from build123d import *

# Parameters (mm, degrees)
EXTRUDE_1_DEPTH     = 4
SKETCH_3_R          = 1.525
CUT_EXTRUDE_3_DEPTH = 5
SKETCH_6_R          = 9.5
CUT_EXTRUDE_5_DEPTH = 5
FILLET_1_R          = 3
SKETCH_7_R          = 1.525
CUT_EXTRUDE_6_DEPTH = 10
CUT_EXTRUDE_7_DEPTH = 10
FILLET_2_R          = 1


with BuildPart() as part:
    # 草图1 → 凸台-拉伸1 (new body)
    with BuildSketch(Plane(origin=(0, 0, 0), x_dir=(1, 0, 0), z_dir=(0, 1, 0))):
        with BuildLine():
            ThreePointArc((-22.5, 20), (-42.5, 0), (-22.5, -20))
            Line((-22.5, -20), (-22.5, 20))
        make_face()
        with BuildLine():
            Line((-22.5, 20), (-22.5, -20))
            ThreePointArc((-22.5, -20), (-8.357864376, -14.142135624), (-2.5, 0))
            ThreePointArc((-2.5, 0), (-8.357864376, 14.142135624), (-22.5, 20))
        make_face()
        with BuildLine():
            ThreePointArc((-2.5, 0), (-8.357864376, -14.142135624), (-22.5, -20))
            Line((-22.5, -20), (22.5, -20))
            Line((22.5, -20), (22.5, 20))
            Line((22.5, 20), (-22.5, 20))
            ThreePointArc((-22.5, 20), (-8.357864376, 14.142135624), (-2.5, 0))
        make_face()
    extrude(amount=EXTRUDE_1_DEPTH)

    # 草图3 → 切除-拉伸3 (cut, through all)
    with BuildSketch(Plane(origin=(0, 0, 0), x_dir=(1, 0, 0), z_dir=(0, 1, 0))):
        with Locations((-36, 0)):
            Circle(SKETCH_3_R)
        with Locations((-29.25, 11.691342951)):
            Circle(SKETCH_3_R)
        with Locations((-15.75, 11.691342951)):
            Circle(SKETCH_3_R)
        with Locations((-9, 0)):
            Circle(SKETCH_3_R)
        with Locations((-15.75, -11.691342951)):
            Circle(SKETCH_3_R)
        with Locations((-29.25, -11.691342951)):
            Circle(SKETCH_3_R)
    extrude(amount=CUT_EXTRUDE_3_DEPTH, mode=Mode.SUBTRACT)

    # 草图6 → 切除-拉伸5 (cut, through all)
    with BuildSketch(Plane.XZ):
        with Locations((-22.5, 0)):
            Circle(SKETCH_6_R)
    extrude(amount=-CUT_EXTRUDE_5_DEPTH, mode=Mode.SUBTRACT)

    # 圆角1
    fillet_1_edges = [part.edges().sort_by_distance(p)[0] for p in [
        (22.5, 2, -20),
        (22.5, 2, 20),
    ]]
    fillet(fillet_1_edges, radius=FILLET_1_R)

    # 草图7 → 切除-拉伸6 (cut)
    with BuildSketch(Plane(origin=(0, 4, 0), x_dir=(1, 0, 0), z_dir=(0, 1, 0))):
        with Locations((19, -14)):
            Circle(SKETCH_7_R)
        with Locations((18.999999998, 13.999999998)):
            Circle(SKETCH_7_R)
    extrude(amount=-CUT_EXTRUDE_6_DEPTH, mode=Mode.SUBTRACT)

    # 草图8 → 切除-拉伸7 (cut)
    with BuildSketch(Plane.XZ):
        with BuildLine():
            Line((-2.5, 4), (12.5, 4))
            Line((12.5, 4), (12.5, 12))
            Line((12.5, 12), (0.5, 12))
            ThreePointArc((0.5, 12), (-0.274661673, 7.727998127), (-2.5, 4))
        make_face()
        with BuildLine():
            Line((12.5, -12), (0.5, -12))
            ThreePointArc((0.5, -12), (-0.274661673, -7.727998127), (-2.5, -4))
            Line((-2.5, -4), (12.5, -4))
            Line((12.5, -4), (12.5, -12))
        make_face()
    extrude(amount=-CUT_EXTRUDE_7_DEPTH, mode=Mode.SUBTRACT)

    # 圆角2
    fillet_2_edges = [part.edges().sort_by_distance(p)[0] for p in [
        (-2.5, 2, 4),
        (0.5, 2, 12),
        (12.5, 2, 12),
        (12.5, 2, 4),
        (0.5, 2, -12),
        (-2.5, 2, -4),
        (12.5, 2, -4),
        (12.5, 2, -12),
    ]]
    fillet(fillet_2_edges, radius=FILLET_2_R)


solid = part.part
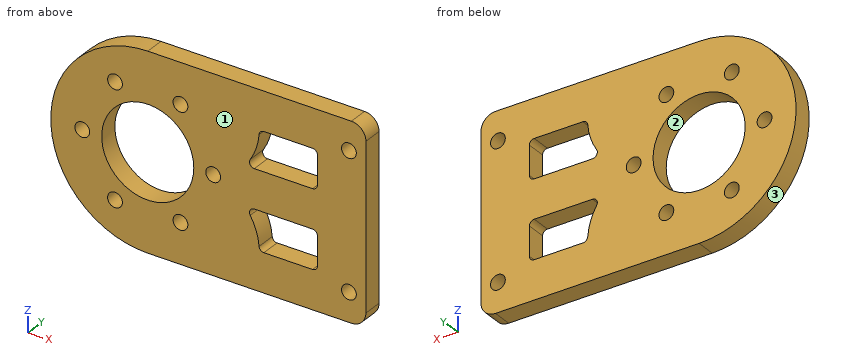
Here's how the part is built. I have some questions about the finished solid (model axes, mm). Face numbers are marked on the shaded views. Give positions to 0.01 mm unless a question says otherwise; leave off trailing zeros. Order: outer loops, then holes, each group sorted by start corner. A loop starts at its lowest first (then second) coordinate and runs counter-clockwise, first axis right, second up. Notation, with made-up numbers: M 57,-11 L 69,-11 A18 cw 69,20 Z; hole C 11,42.25 d7. An arc over 180 degrees is marked long. Answer as a JSON object with one key per item and string values. Group by question number.
1) We'd pull the mould along Z, two halves only. Please class the marked faces 1, 2 and 3: pulls with the +Z half, pulls with the -Z half, needs draft (parallel to the pull), parting line crosses it, or undercut.
2) Please list where these lines run through material, in increasing order: L1, parallel to Z at x = 5, y = 3.2; L2, parallel to Z at x = 19, y = 2.7 (3 decimals); L3, parallel to Z at x = -15.5, y = 1.15. Write a range as [from, to].
3) Suppose I cut it at C-C, the plane x = 2.5. Write out the boundary of the cut face in (y, z), plus the area to 3 significant figures.
4) Suppose I cut it at A-A, the plane x = -9. Write out the boundary of the cut face in (y, z) (3 decimals), plus the area to 3 significant figures.
5) Suppose I cut it at D-D, the plane y = 1. Count the separate pieces of the cut face and the enclosed holes in it, plus the area to 3 significant figures.
6) Suppose I cut it at B-B, the plane z = 0. Write out the boundary of the cut face in (x, y) (3 decimals).
7) I'm going to push flat-ended pins straight in: pin 1 Ø1.2 at (y, z) = (1.5, 7) entering from -X; pin 2 Ø1.5 at (y, z) = (1, 1) entering from -X. Where does each tip first touch, or does it pass through?
Results found:
{
 "1": {"face 1": "needs draft", "face 2": "undercut", "face 3": "parting line crosses it"},
 "2": {"L1": "[-20, -12], [-4, 4], [12, 20]", "L2": "[-20, -15.525], [-12.475, 12.475], [15.525, 20]", "L3": "[-20, -13.2], [-10.19, -6.42], [6.42, 10.19], [13.2, 20]"},
 "3": {"outline": "M 0,-20 L 4,-20 L 4,-12 L 0,-12 Z; M 0,-4 L 4,-4 L 4,4 L 0,4 Z; M 0,12 L 4,12 L 4,20 L 0,20 Z", "area": "96.0 mm²"},
 "4": {"outline": "M 0,-20 L 4,-20 L 4,-1.525 L 0,-1.525 Z; M 0,1.525 L 4,1.525 L 4,20 L 0,20 Z", "area": "148 mm²"},
 "5": {"separate pieces": "1", "enclosed holes": "11", "area": "1,880 mm²"},
 "6": {"outline": "M -42.5,0 L -37.525,0 L -37.525,4 L -42.5,4 Z; M -34.475,0 L -32,0 L -32,4 L -34.475,4 Z; M -13,0 L -10.525,0 L -10.525,4 L -13,4 Z; M -7.475,0 L 22.5,0 L 22.5,4 L -7.475,4 Z"},
 "7": {"pin 1": "x = -41.45", "pin 2": "x = -42.5"}
}
